```python
from build123d import *

# Parameters (mm, degrees)
BOSS_EXTRUDE1_DEPTH = 10
CUT_EXTRUDE1_DEPTH  = 3


with BuildPart() as part:
    # Sketch1 → Boss-Extrude1 (new body)
    with BuildSketch(Plane.XY):
        with BuildLine():
            ThreePointArc((18.5, 0), (-1.504988227, -18.438682449), (-18.255136264, 3))
            Line((-18.255136264, 3), (-28.255136264, 3))
            Line((-28.255136264, 3), (-28.255136264, 0))
            Line((-28.255136264, 0), (-21.5, 0))
            ThreePointArc((-21.5, 0), (0, -21.5), (21.5, 0))
            Line((21.5, 0), (28.255136264, 0))
            Line((28.255136264, 0), (28.255136264, 3))
            Line((28.255136264, 3), (18.255136264, 3))
            ThreePointArc((18.255136264, 3), (18.438682449, 1.504988227), (18.5, 0))
        make_face()
    extrude(amount=BOSS_EXTRUDE1_DEPTH)

    # Sketch2 → Cut-Extrude1 (cut)
    with BuildSketch(Plane(origin=(0, 3, 0), x_dir=(1, 0, 0), z_dir=(0, 1, 0))):
        with BuildLine():
            ThreePointArc((-23.255136264, -5), (-24.755136264, -3.5), (-26.255136264, -5))
            Line((-26.255136264, -5), (-23.255136264, -5))
        make_face()
        with BuildLine():
            Line((-23.255136264, -5), (-26.255136264, -5))
            ThreePointArc((-26.255136264, -5), (-24.755136264, -6.5), (-23.255136264, -5))
        make_face()
    cut_extrude1 = extrude(amount=-CUT_EXTRUDE1_DEPTH, mode=Mode.SUBTRACT)

    # Mirror1: Cut-Extrude1 across plane
    add(cut_extrude1.mirror(Plane(origin=(0, 0, 0), x_dir=(0, 0, 1), z_dir=(1, 0, 0))), mode=Mode.SUBTRACT)


solid = part.part
```
The listing builds one solid part. Answer for the finished solid, in the listing's coordinates (mm). A direction names the side the tool comes from. Give positions to 0.01 mm unless a question says otherwise; leave off trailing zeros. Write each loop counter-clockwise with the first axis right and the second up, starting at its lowest first coordinate (ties: lowest second). Pieces come first, ordered by that corner, then holes. Notation, with made-up numbers: (-37, 52) -> (4, 52) arc R29 ccw to (4, 86) -> close; hole circle Ø2 at (43, -30.5). An arc over 180 degrees is marked (long way). Write item = value, one per line. Start each with the question number.
1) The part is cut by section B-B, the plane y = 1.75. Determine the outline of the cut face in (x, z).
2) The part is cut by section D-D, the plane y = -7.25. Determine the outline of the cut face in (x, z).
3) Each of these flat-tipped pins is pushed along its axis until it touches: pin 1 (1.5 mm diameter, centred on y = -13, z = 2.5, fed in from +X); pin 2 (1.5 mm diameter, centred on x = 17.5, z = 5.5, fed in from -Y); pin 3 (2 mm diameter, centred on x = 17, y = -6.5, fed in from +Z); pin 4 (2.5 mm diameter, centred on x = 24.76, z = 5, fed in from +Y). Where does it stop, or does it pass through?
4) Determine the mould class of faces 1 (the face through (-23, 3, 5)), 2 (the face through (4.1, -18.3, 10)), 3 (the face through (23.257, 1.521, 5.066)) for opening direction Z: +Z half, -Z half, draft (parallel to the pull), parting line (faces both ways), or undercut.
5) Straight lines are drawn through the part: line 1 along Y through (x, z) = (0, 2); line 2 along X through (y, z) = (0.5, 3.75); line 3 along X through (y, z) = (-3.5, 2). For each, find the intervals that lie inside material, in ascending order.
6) Which of the six approach directions +Z, -Z, +X, -X, +Y, -Y give full straight-line access (tool end or side, diameter ignored) to faces 4 (the face through (26.3, 0, 3.8)), 5 (the face through (4.1, -18.3, 0)), 6 (the face through (-26.43, 0, 4.93))?
7) The part is cut by section A-A, the plane z = 5. Determine the outline of the cut face in (x, y), and give its area (3 significant figures).
8) The part is cut by section C-C, the plane z = 8. Determine the outline of the cut face in (x, y).
Solutions:
q1.outline = (-28.26, 0) -> (-18.42, 0) -> (-18.42, 10) -> (-28.26, 10) -> close; (18.42, 0) -> (28.26, 0) -> (28.26, 10) -> (18.42, 10) -> close; hole circle Ø3 at (-24.76, 5); hole circle Ø3 at (24.76, 5)
q2.outline = (-20.24, 0) -> (-17.02, 0) -> (-17.02, 10) -> (-20.24, 10) -> close; (17.02, 0) -> (20.24, 0) -> (20.24, 10) -> (17.02, 10) -> close
q3.pin_1 = 17.67
q3.pin_2 = -13.48
q3.pin_3 = 10
q3.pin_4 = through
q4.face_1 = draft
q4.face_2 = +Z half
q4.face_3 = undercut
q5.line_1 = -21.5 to -18.5
q5.line_2 = -28.26 to -25.58, -23.93 to -18.49, 18.49 to 23.93, 25.58 to 28.26
q5.line_3 = -21.21 to -18.17, 18.17 to 21.21
q6.face_4 = +Z, -Z, +X, -Y
q6.face_5 = -Z, +X, -X, +Y, -Y
q6.face_6 = +Z, -Z, -X, -Y
q7.outline = (-28.26, 0) -> (-26.26, 0) -> (-26.26, 3) -> (-28.26, 3) -> close; (-23.26, 0) -> (-21.5, 0) arc R21.5 ccw to (21.5, 0) -> (23.26, 0) -> (23.26, 3) -> (18.26, 3) arc R18.5 cw (long way) to (-18.26, 3) -> (-23.26, 3) -> close; (26.26, 0) -> (28.26, 0) -> (28.26, 3) -> (26.26, 3) -> close
q7.area = 230 mm²
q8.outline = (-28.26, 0) -> (-21.5, 0) arc R21.5 ccw to (21.5, 0) -> (28.26, 0) -> (28.26, 3) -> (18.26, 3) arc R18.5 cw (long way) to (-18.26, 3) -> (-28.26, 3) -> close
